Autodesk Inventor part; units mm, degrees
ref_plane "YZ Plane" through (0, 0, 0) normal (1, 0, 0) x (0, 1, 0)
ref_plane "XZ Plane" through (0, 0, 0) normal (0, 1, 0) x (-1, 0, 0)
ref_plane "XY Plane" through (0, 0, 0) normal (0, 0, 1) x (1, 0, 0)
sketch "Sketch1" plane through (0, 0, 0) normal (0, 1, 0) x (-1, 0, 0)
  line L0 (0, 0) -> (431.8, 0)
  line L1 (431.8, 0) -> (431.8, 431.8)
  line L2 (431.8, 431.8) -> (0, 431.8)
  line L3 (0, 431.8) -> (0, 0)
  dimension "d0" = 431.8
  dimension "d2" = 431.8
extrude "Extrusion1" add sketch "Sketch1" along normal blind 3.175
sketch "Sketch2" plane through (0, 3.175, 0) normal (0, 1, 0) x (1, 0, 0)
  line L0 (0, 0) -> (-431.8, 0)
  line L1 (-431.8, 0) -> (-431.8, -431.8)
  line L2 (-431.8, -431.8) -> (0, -431.8)
  line L3 (0, -431.8) -> (0, 0)
  line L4 (-257.175, -114.3) -> (-174.625, -114.3)
  line L5 (-174.625, -114.3) -> (-174.625, -19.05)
  line L6 (-257.175, -31.75) -> (-257.175, -114.3)
  line L7 (0, -215.9) -> (-431.8, -215.9)
  line L8 (-174.625, 0) -> (-174.625, -19.05)
  line L9 (-257.175, -31.75) -> (-257.175, 0)
  line L10 (-215.9, -431.8) -> (-215.9, -215.9)
  dimension "d5" = 82.55
  dimension "d7" = 82.55
  dimension "d8" = 215.9
  dimension "d9" = 101.6
  dimension "d10" = 41.275
  dimension "d51" = 174.625
  dimension "d52" = 174.625
extrude "Extrusion2" cut sketch "Sketch2" against normal blind 3.175 contours L8 L5 L4 L6 L9 L0
sketch "Sketch3" plane through (0, 3.175, 0) normal (0, 1, 0) x (1, 0, 0)
  line L0 (-431.8, 0) -> (-431.8, -431.8)
  line L1 (-431.8, -431.8) -> (0, -431.8)
  line L2 (-266.7, -268.7828) -> (-165.1, -268.7828)
  line L3 (-165.1, -268.7828) -> (-165.1, -167.1828)
  line L4 (-165.1, -167.1828) -> (-266.7, -167.1828)
  line L5 (-266.7, -167.1828) -> (-266.7, -268.7828)
  line L6 (-215.9, -167.1828) -> (-215.9, -268.7828)
  line L7 (-165.1, -217.9828) -> (-266.7, -217.9828)
  line L8 (0, -431.8) -> (0, 0)
  dimension "d13" = 101.6
  dimension "d15" = 101.6
  dimension "d18" = 215.9
  dimension "d19" = 213.8172
  dimension "d55" = 50.8
  dimension "d56" = 50.8
  dimension "d57" = 215.9
hole "Hole1" at (-165.1, 3.175, 167.1828) at (-266.7, 3.175, 217.9828) at (-266.7, 3.175, 268.7828) at (-165.1, 3.175, 268.7828) direction (0, -1, 0) diameter 6.35 end through all
sketch "Sketch4" plane through (0, 3.175, 0) normal (0, 1, 0) x (1, 0, 0)
  circle A0 centre (-165.1, -167.1828) radius 3.175
  circle A1 centre (-266.7, -217.9828) radius 3.175
  circle A2 centre (-165.1, -268.7828) radius 3.175
  line L0 (-254, -268.7828) -> (-180.975, -268.7828)
  line L1 (-180.975, -268.7828) -> (-180.975, -179.8828)
  line L2 (-180.975, -179.8828) -> (-254, -179.8828)
  line L3 (-254, -179.8828) -> (-254, -268.7828)
  line L4 (-431.8, 0) -> (-431.8, -431.8)
  line L5 (0, -431.8) -> (0, 0)
  dimension "d27" = 12.7
  dimension "d28" = 12.7
  dimension "d29" = 12.7
  dimension "d30" = 88.9
  dimension "d53" = 177.8
  dimension "d54" = 180.975
extrude "Extrusion3" cut sketch "Sketch4" against normal blind 3.175 contours L3 L2 L1 L0
sketch "Sketch5" plane through (0, 3.175, 0) normal (0, 1, 0) x (1, 0, 0)
  line L0 (-431.8, 0) -> (-431.8, -431.8)
  line L1 (-431.8, -431.8) -> (0, -431.8)
  line L2 (0, -431.8) -> (0, 0)
  point P0 (-419.1, -215.9)
  point P1 (-215.9, -419.1)
  point P2 (-12.7, -215.9)
  dimension "d33" = 12.7
  dimension "d34" = 12.7
  dimension "d35" = 12.7
  dimension "d36" = 215.9
  dimension "d37" = 215.9
  dimension "d38" = 215.9
hole "Hole2" at (-419.1, 3.175, 215.9) at (-215.9, 3.175, 419.1) at (-12.7, 3.175, 215.9) direction (0, -1, 0) diameter 6.35 end through all
sketch "Sketch6" plane through (0, 3.175, 0) normal (0, 1, 0) x (1, 0, 0)
  line L0 (0, -431.8) -> (0, 0)
  line L1 (0, 0) -> (-174.625, 0)
  line L2 (-174.625, 0) -> (-174.625, -114.3)
  line L3 (-174.625, -12.7) -> (0, -12.7)
  dimension "d46" = 12.7
extrude "Extrusion4" cut sketch "Sketch6" against normal blind 25.4
sketch "Sketch7" plane through (0, 3.175, 0) normal (0, 1, 0) x (1, 0, 0)
  line L0 (-257.175, -114.3) -> (-257.175, 0)
  line L1 (-257.175, 0) -> (-431.8, 0)
  line L2 (-431.8, 0) -> (-431.8, -431.8)
  line L3 (-257.175, -12.7) -> (-431.8, -12.7)
  point P0 (0, 0)
  dimension "d58" = 12.7
extrude "Extrusion5" cut sketch "Sketch7" against normal blind 25.4
sketch "Sketch8" plane through (0, 3.175, 0) normal (0, 1, 0) x (1, 0, 0)
  line L0 (-257.175, -12.7) -> (-431.8, -12.7)
  line L1 (-431.8, -12.7) -> (-431.8, -431.8)
  line L2 (-431.8, -431.8) -> (0, -431.8)
  line L3 (0, -431.8) -> (0, -12.7)
  line L4 (0, -12.7) -> (-174.625, -12.7)
  point P0 (0, 0)
  point P1 (-419.1, -25.4)
  point P2 (-12.7, -25.4)
  point P3 (-419.1, -419.1)
  point P4 (-12.7, -419.1)
  dimension "d59" = 12.7
  dimension "d60" = 12.7
  dimension "d61" = 12.7
  dimension "d62" = 12.7
  dimension "d63" = 12.7
  dimension "d64" = 12.7
  dimension "d65" = 12.7
  dimension "d66" = 12.7
hole "Hole3" at (-419.1, 3.175, 25.4) at (-12.7, 3.175, 25.4) at (-419.1, 3.175, 419.1) at (-12.7, 3.175, 419.1) direction (0, -1, 0) diameter 6.35 end through all
sketch "Sketch9" plane through (0, 0, 0) normal (0, -1, 0) x (1, 0, 0)
  line L0 (0, 431.8) -> (0, 12.7)
  point P0 (0, 0)
  point P1 (-34.29, 134.8443)
  dimension "d74" = 34.29
hole "Hole4" at (-34.29, 0, 134.8443) direction (0, 1, 0) diameter 3 end through all
sketch "Sketch10" plane through (0, 0, 0) normal (0, -1, 0) x (1, 0, 0)
  line L0 (0, 431.8) -> (0, 12.7)
  point P0 (0, 0)
  point P1 (-31.75, 281.1231)
  dimension "d82" = 31.75
hole "Hole5" at (-31.75, 0, 281.1231) direction (0, 1, 0) diameter 3 end through all
sketch "Sketch12" plane through (0, 0, 0) normal (0, -1, 0) x (1, 0, 0)
  circle A0 centre (-34.29, 134.8443) radius 1.5
  line L0 (0, 431.8) -> (0, 12.7)
  line L1 (-34.29, 134.8443) -> (-50.0054, 119.1289)
  line L2 (-50.0054, 119.1289) -> (-42.7314, 111.8548)
  point P0 (0, 0)
  dimension "d108" = 45
  dimension "d109" = 22.225
  dimension "d110" = 10.287
hole "Hole7" at (-42.7314, 0, 111.8548) direction (0, 1, 0) diameter 3 depth 25.4 tip angle 118
sketch "Sketch13" plane through (0, 0, 0) normal (0, -1, 0) x (1, 0, 0)
  circle A0 centre (-31.75, 281.1231) radius 1.5
  line L0 (0, 431.8) -> (0, 12.7)
  line L1 (-31.75, 281.1231) -> (-30.1997, 258.9522)
  line L2 (-30.1997, 258.9522) -> (-19.9377, 259.6698)
  point P0 (0, 0)
  dimension "d118" = 4
  dimension "d119" = 22.225
  dimension "d120" = 10.287
hole "Hole8" at (-19.9377, 0, 259.6698) direction (0, 1, 0) diameter 3 depth 25.4 tip angle 118
properties part number "New BottomHopper Plate" material "Aluminum 6061"
Check sheet for the modelled part. Datum: model origin and axes. Units: mm. Round coordinates to 2 decimals unless told otherwise and drop trailing zeros. Order: outer loops, then holes, each group sorted by start corner. A loop starts at its lowest first (then second) coordinate and runs counter-clockwise, first axis right, second up. Notation, with made-up numbers: (-25, -10.5) -> (34, -10.5) arc R29 ccw to (34, 17.5) -> close; hole circle Ø5 at (72, 74.5). An arc over 180 degrees is marked (long way). Use CSV: the item, a comma, the result in double quotes.
(1) Cross-section at B-B (z = 46). Record the boundary of the cut face in (x, y) (3 decimals).
Worked out:
outline,"(-431.8, 0) -> (-257.175, 0) -> (-257.175, 3.175) -> (-431.8, 3.175) -> close; (-174.625, 0) -> (0, 0) -> (0, 3.175) -> (-174.625, 3.175) -> close"
(2) Material ranges on line 1 along X through (y, z) = (2.45, 419.1) (3 decimals); line 2 along Z through (x, y) = (-165.1, 1.35); line 3 along Z through (x, y) = (-43, 1.25), recorded low to high. Write a range as from..to.
Worked out:
line 1,"-431.8..-422.275, -415.925..-219.075, -212.725..-15.875, -9.525..0"
line 2,"12.7..164.01, 170.36..265.61, 271.96..431.8"
line 3,"12.7..110.38, 113.33..431.8"
(3) Depth check by flat-ended pin: pin 1 (1.5 mm diameter, centred on y = 2, z = 204, fed in from +X); pin 2 (4 mm diameter, centred on x = -266.7, z = 268.78, fed in from +Y). Enter the tip coordinate at first touch or a pass-through.
Worked out:
pin 1,"x = 0"
pin 2,"through"
(4) Cross-section at C-C (y = 0.7). Count the separate pieces of the cut face and the enclosed holes in it, and give its area (3 significant figures).
Worked out:
separate pieces,"1"
enclosed holes,"16"
area,"166,000 mm²"
(5) Cross-section at A-A (x = -234.5). Record the boundary of the cut face in (y, z) (3 decimals).
Worked out:
outline,"(0, 114.3) -> (3.175, 114.3) -> (3.175, 179.883) -> (0, 179.883) -> close; (0, 268.783) -> (3.175, 268.783) -> (3.175, 431.8) -> (0, 431.8) -> close"
